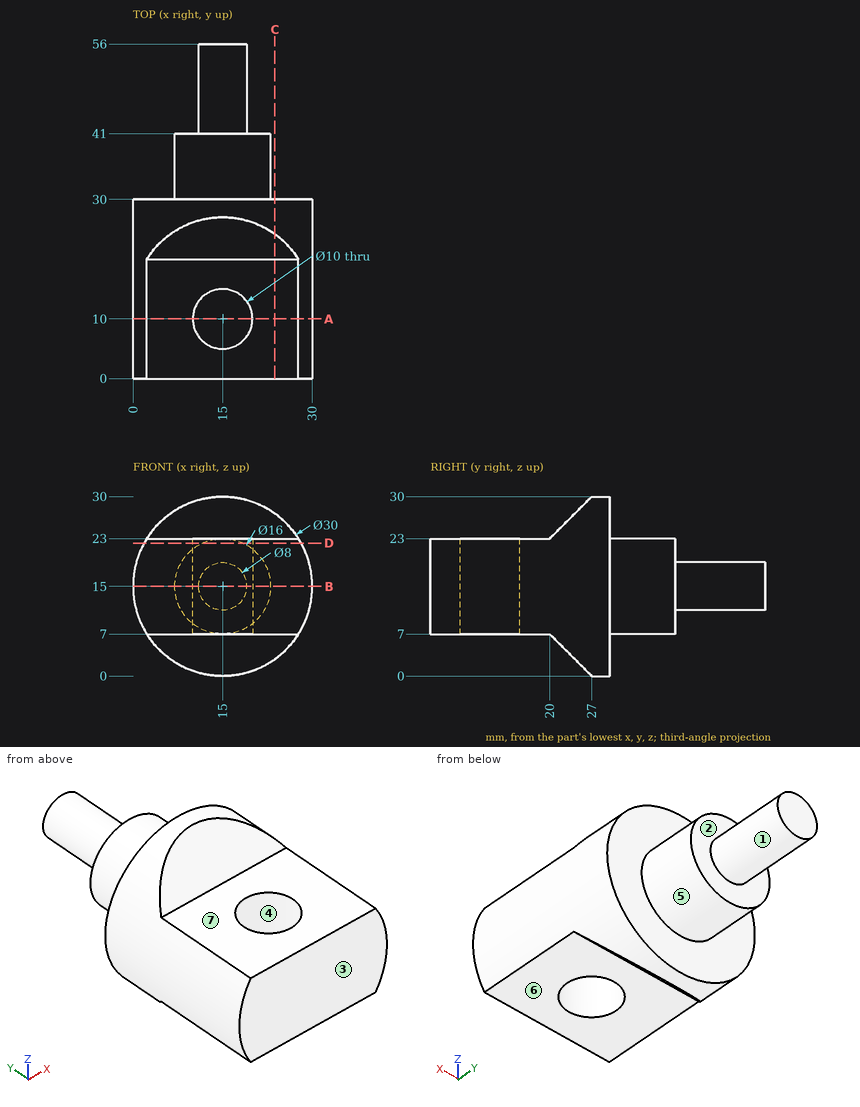
Answer from the drawing. Dimensions are ordinates in mm from the lowest x, y and z of the part. A direction names the side the tool comes from. Give positions to 0.01 mm unless a question says otherwise; leave off trailing zeros. Order: outer loops, then holes, each group sorted by start corner. A loop starts at its lowest first (then second) coordinate and runs counter-clockwise, first axis right, second up. Notation, with made-up numbers: (-32.5, -2) - (0.5, -2) arc R16 ccw to (0.5, 5) - close; hole circle Ø2 at (52.5, 26). An arc over 180 degrees is marked (long way). One line per item, written item: value. Start each with the question number.
1. Consider line 1 (Y direction, x = 15, z = 14); line 2 (Z direction, x = 24.75, y = 18.5); line 3 (Y direction, x = 25, z = 17.5). Determine where each line is inside the solid, lowest interval first.
2. Each of these flat-tipped pins is pushed along its axis until it touches: pin 1 Ø2 at (y, z) = (8, 13) entering from -X; pin 2 Ø3 at (x, z) = (25, 20) entering from +Y; pin 3 Ø3 at (x, y) = (7, 30) entering from -Z; pin 4 Ø8 at (x, z) = (13, 10) entering from -Y. Where does it stop, or does it pass through?
3. Which of the six approach directions +Z, -Z, +X, -X, +Y, -Y give full straight-line access (tool end or side, diameter ignored) to the marked faces 5, 6 and 7?
4. Section D-D, the plane z = 22.25 is taken. Write down the section's boundary in (x, y).
5. Section A-A, the plane y = 10 is taken. Write down the section's boundary in (x, z).
6. Section C-C, the plane x = 23.75 is taken. Write down the section's boundary in (y, z).
7. Section B-B, the plane z = 15 is taken. Write down the section's boundary in (x, y), then the cut area to 3 significant figures.
8. For a pull along Y with two mould halves and no side action, classify the marked faces 1, 2, 3 and 4 as released by +Y, released by -Y, zero draft, split by the parting line, or undercut.
Filled sheet:
1. line 1: 0 to 5, 15 to 56
1. line 2: 7 to 23
1. line 3: 0 to 30
2. pin 1: x = 0.03
2. pin 2: y = 30
2. pin 3: z = 1.48
2. pin 4: y = 0
3. face 5: +Y
3. face 6: -Z, +X, -X, -Y
3. face 7: +Z, +X, -X, -Y
4. outline: (1.87, 0) - (28.13, 0) - (28.13, 30) - (18.38, 30) - (18.38, 41) - (11.62, 41) - (11.62, 30) - (1.87, 30) - close; hole circle Ø10 at (15, 10)
5. outline: (2.31, 7) - (10, 7) - (10, 23) - (2.31, 23) arc R15 ccw to start; (20, 7) - (27.69, 7) arc R15 ccw to (27.69, 23) - (20, 23) - close
6. outline: (0, 7) - (20, 7) - (24.18, 2.82) - (30, 2.82) - (30, 27.18) - (24.18, 27.18) - (20, 23) - (0, 23) - close
7. outline: (0, 0) - (30, 0) - (30, 30) - (23, 30) - (23, 41) - (19, 41) - (19, 56) - (11, 56) - (11, 41) - (7, 41) - (7, 30) - (0, 30) - close; hole circle Ø10 at (15, 10)
7. area: 1,120 mm²
8. face 1: zero draft
8. face 2: released by +Y
8. face 3: released by -Y
8. face 4: undercut
